Build history of the part. All positions in model axes, mm. Face numbers are marked on the shaded views. A direction names the side the tool comes from. Coordinates: 2 decimals unless noted, no trailing zeros. Order: outer loops, then holes, each group sorted by start corner. A loop starts at its lowest first (then second) coordinate and runs counter-clockwise, first axis right, second up. Notation, with made-up numbers: M 50.25,56 L 58.25,56 A23 ccw 58.25,84 Z; hole C 62,53 d11. An arc over 180 degrees is marked long. Use a Markdown table: item, result. Add a question column.
from build123d import *

# Parameters (mm, degrees)
SKETCH_2_W                = 40
SKETCH_2_H                = 39
EXTRUDE_1_DEPTH           = 10
FILLET_1_R                = 1
SKETCH_6_R                = 4
CUT_EXTRUDE_1_DEPTH       = 2
HOLE_WIZARD_2_0_2_2_D     = 2
HOLE_WIZARD_2_0_2_2_DEPTH = 10
HOLE_WIZARD_2_0_2_2_TIP   = 0.600860619
EXTRUDE_START             = -8
SKETCH_16_W               = 7
SKETCH_16_H               = 19
SKETCH_16_R               = 2
EXTRUDE_2_DEPTH           = 3
SKETCH_17_R               = 6.5
EXTRUDE_3_DEPTH           = 1.5
SKETCH_18_R               = 5
EXTRUDE_4_DEPTH           = 0.5
SKETCH_19_R               = 3
EXTRUDE_5_DEPTH           = 4
FILLET_2_R                = 1
HOLE_WIZARD_M3_1_D        = 2.5
HOLE_WIZARD_M3_1_DEPTH    = 5.55
HOLE_WIZARD_M3_1_TIP      = 0.751075774


with BuildPart() as part:
    # 草图2 → 凸台-拉伸1 (new, symmetric)
    with BuildSketch(Plane.XY):
        with Locations((20, -19.5)):
            Rectangle(SKETCH_2_W, SKETCH_2_H)
    extrude(amount=EXTRUDE_1_DEPTH, both=True)

    # 圆角1
    fillet_1_edges = [part.edges().sort_by_distance(p)[0] for p in [
        (40, -19.5, 10),
        (20, 0, 10),
        (0, -19.5, 10),
        (20, 0, -10),
        (40, -19.5, -10),
        (20, -39, -10),
        (0, -19.5, -10),
        (20, -39, 10),
        (0, 0, 0),
        (40, 0, 0),
        (40, -39, 0),
        (0, -39, 0),
    ]]
    fillet(fillet_1_edges, radius=FILLET_1_R)

    # 草图6 → 切除-拉伸1 (cut)
    with BuildSketch(Plane.XZ):
        with Locations((0, 10)):
            Circle(SKETCH_6_R)
        with Locations((40, 10)):
            Circle(SKETCH_6_R)
        with Locations((40, -10)):
            Circle(SKETCH_6_R)
        with Locations((0, -10)):
            Circle(SKETCH_6_R)
    extrude(amount=CUT_EXTRUDE_1_DEPTH, mode=Mode.SUBTRACT)

    # Ø2.0 (2) 直径孔2
    with Locations(Plane(origin=(0, -39, 0), x_dir=(-1, 0, 0), z_dir=(0, -1, 0))):
        with Locations((-37.5, 7.5), (-37.5, -7.5), (-2.5, 7.5), (-2.5, -7.5)):
            Hole(HOLE_WIZARD_2_0_2_2_D / 2, depth=HOLE_WIZARD_2_0_2_2_DEPTH)
            with Locations((0, 0, -(HOLE_WIZARD_2_0_2_2_DEPTH + HOLE_WIZARD_2_0_2_2_TIP / 2))):  # 118° drill point
                Cone(0, HOLE_WIZARD_2_0_2_2_D / 2, HOLE_WIZARD_2_0_2_2_TIP, mode=Mode.SUBTRACT)

    # 草图16 → 凸台-拉伸2 (add)
    # profile 1 of 2: a face of its own
    with BuildSketch(Plane(origin=(0, 0, 0), x_dir=(1, 0, 0), z_dir=(0, 1, 0)).offset(EXTRUDE_START)):
        with Locations((-3.5, 0)):
            Rectangle(SKETCH_16_W, SKETCH_16_H)
        with Locations(Location((-4, -5, 0), (0, 0, 270))):
            Circle(SKETCH_16_R, mode=Mode.SUBTRACT)
        with Locations(Location((-4, 5, 0), (0, 0, 270))):
            Circle(SKETCH_16_R, mode=Mode.SUBTRACT)
    # profile 2 of 2: a face of its own
    with BuildSketch(Plane(origin=(0, 0, 0), x_dir=(1, 0, 0), z_dir=(0, 1, 0)).offset(EXTRUDE_START)):
        with Locations((43.5, 0)):
            Rectangle(SKETCH_16_W, SKETCH_16_H)
        with Locations(Location((44, 5, 0), (0, 0, 90))):
            Circle(SKETCH_16_R, mode=Mode.SUBTRACT)
        with Locations(Location((44, -5, 0), (0, 0, 90))):
            Circle(SKETCH_16_R, mode=Mode.SUBTRACT)
    extrude(amount=-EXTRUDE_2_DEPTH)

    # 草图17 → 凸台-拉伸3 (add)
    with BuildSketch(Plane(origin=(0, 0, 0), x_dir=(1, 0, 0), z_dir=(0, 1, 0))):
        with Locations(Location((10, 0, 0), (0, 0, 90))):
            Circle(SKETCH_17_R)
    extrude(amount=EXTRUDE_3_DEPTH)

    # 草图18 → 凸台-拉伸4 (add)
    with BuildSketch(Plane(origin=(0, 1.5, 0), x_dir=(1, 0, 0), z_dir=(0, 1, 0))):
        with Locations(Location((10, 0, 0), (0, 0, 270))):
            Circle(SKETCH_18_R)
    extrude(amount=EXTRUDE_4_DEPTH)

    # 草图19 → 凸台-拉伸5 (add)
    with BuildSketch(Plane(origin=(0, 2, 0), x_dir=(1, 0, 0), z_dir=(0, 1, 0))):
        with Locations(Location((10, 0, 0), (0, 0, 270))):
            Circle(SKETCH_19_R)
    extrude(amount=EXTRUDE_5_DEPTH)

    # 圆角2
    fillet_2_edges = [part.edges().sort_by_distance(p)[0] for p in [
        (-7, -9.5, 9.5),
        (-7, -9.5, -9.5),
        (47, -9.5, 9.5),
        (47, -9.5, -9.5),
    ]]
    fillet(fillet_2_edges, radius=FILLET_2_R)

    # M3 螺纹孔1
    with Locations(Plane(origin=(0, 6, 0), x_dir=(1, 0, 0), z_dir=(0, 1, 0))):
        with Locations((10, 0)):
            Hole(HOLE_WIZARD_M3_1_D / 2, depth=HOLE_WIZARD_M3_1_DEPTH)
            with Locations((0, 0, -(HOLE_WIZARD_M3_1_DEPTH + HOLE_WIZARD_M3_1_TIP / 2))):  # 118° drill point
                Cone(0, HOLE_WIZARD_M3_1_D / 2, HOLE_WIZARD_M3_1_TIP, mode=Mode.SUBTRACT)


solid = part.part
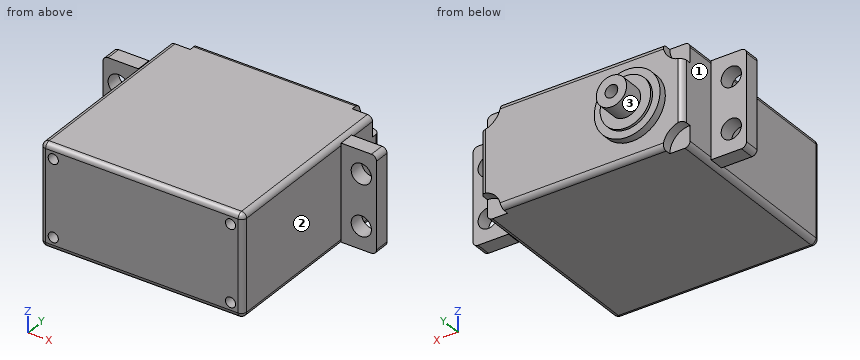
(1) Slice it at B-B on x = 44. Give the cut face in (y, z), and give its area (3 significant figures).
(2) Slice it at A-A on y = -34. Give the cut face in (x, z), and give its area (3 significant figures).
(3) Slice it at D-D on y = -26. Give the cut face in (x, z).
(4) Drop flat-ended pins along their axis: P1, Ø1, axis at y = -3, z = 2.5, coming from the +X side; P2, Ø5.5, axis at x = 44, z = -4.5, coming from the +Y side; P3, Ø3.5, axis at y = -3.5, z = -2, coming from the -X side; P4, Ø3, axis at x = -4, z = 5, coming from the -Y side. Give the stop position or say it passes through.
(5) Drill centre lines: line 1 along X through (y, z) = (-10.2, -5); line 2 along Z through (x, y) = (2.5, -33); line 3 along X through (y, z) = (-36.25, 7.5). Where is each one in solid material? Low to high. Write a range as from..to.
(6) Which spindle directions (+Z, -Z, +X, -X, +Y, -Y) get a long thin tool onto all of the face, cutting with end or side? Do the marked faces 1, 2 and 3. Say none if no direction does.
(7) Slice it at C-C on z = -3.75. State how many separate pieces and enclosed holes the cut face has, and give its area (3 significant figures).
Solutions:
| question | item | result |
|---|---|---|
| 1 | outline | M -11,-9.5 L -8,-9.5 L -8,-7 L -11,-7 Z; M -11,-3 L -8,-3 L -8,3 L -11,3 Z; M -11,7 L -8,7 L -8,9.5 L -11,9.5 Z |
| 1 | area | 33.0 mm² |
| 2 | outline | M 0,-9 A1 ccw 1,-10 L 39,-10 A1 ccw 40,-9 L 40,9 A1 ccw 39,10 L 1,10 A1 ccw 0,9 Z; hole C 2.5,-7.5 d2; hole C 2.5,7.5 d2; hole C 37.5,-7.5 d2; hole C 37.5,7.5 d2 |
| 2 | area | 787 mm² |
| 3 | outline | M 0,-9 A1 ccw 1,-10 L 39,-10 A1 ccw 40,-9 L 40,9 A1 ccw 39,10 L 1,10 A1 ccw 0,9 Z |
| 4 | P1 | x = 40 |
| 4 | P2 | y = -8 |
| 4 | P3 | x = 0 |
| 4 | P4 | through |
| 5 | line 1 | -7..-6, -2..42, 46..47 |
| 5 | line 2 | -10..-8.5, -6.5..6.5, 8.5..10 |
| 5 | line 3 | 0..1.5, 3.5..36.5, 38.5..40 |
| 6 | face 1 | +Z, -Z, -X, +Y |
| 6 | face 2 | +Z, -Z, +X, -Y |
| 6 | face 3 | +Y |
| 7 | separate pieces | 3 |
| 7 | enclosed holes | 0 |
| 7 | area | 1,600 mm² |
